from build123d import *

# Parameters (mm, degrees)
BOSS_EXTRUDE1_DEPTH = 6.35
CUT_EXTRUDE1_DEPTH  = 7.35
SKETCH4_R           = 3
CUT_EXTRUDE2_DEPTH  = 7.35


with BuildPart() as part:
    # Sketch2 → Boss-Extrude1 (new body)
    with BuildSketch(Plane.XY):
        with BuildLine():
            ThreePointArc((-100, 73.02486306), (0, 79.721425695), (100, 73.02486306))
            ThreePointArc((100, 73.02486306), (123.825, 0), (100, -73.02486306))
            ThreePointArc((100, -73.02486306), (0, -79.721425695), (-100, -73.02486306))
            ThreePointArc((-100, -73.02486306), (-123.825, 0), (-100, 73.02486306))
        make_face()
    extrude(amount=BOSS_EXTRUDE1_DEPTH)

    # Sketch3 → Cut-Extrude1 (cut, through all)
    with BuildSketch(Plane.XY.offset(6.35)):
        with BuildLine():
            Line((-61.572799723, 14.542440806), (-81.281148146, 14.542440806))
            ThreePointArc((-81.281148146, 14.542440806), (-91.5900314, 19.825101253), (-93.322799723, 31.278357963))
            ThreePointArc((-93.322799723, 31.278357963), (-87.27608067, 45.501278749), (-79.077484693, 58.602321112))
            ThreePointArc((-79.077484693, 58.602321112), (-75.119328128, 62.098990903), (-70.081085695, 63.683230851))
            ThreePointArc((-70.081085695, 63.683230851), (-59.910981492, 64.583293189), (-49.729388954, 65.342440806))
            ThreePointArc((-49.729388954, 65.342440806), (-40.200680121, 61.949526114), (-36.172799723, 52.671361338))
            Line((-36.172799723, 52.671361338), (-36.172799723, 39.942440806))
            ThreePointArc((-36.172799723, 39.942440806), (-43.612287481, 21.981928564), (-61.572799723, 14.542440806))
        make_face()
        with BuildLine():
            Line((36.172799723, -29.907559194), (36.172799723, -52.671361338))
            ThreePointArc((36.172799723, -52.671361338), (40.200680121, -61.949526114), (49.729388954, -65.342440806))
            ThreePointArc((49.729388954, -65.342440806), (59.910981492, -64.583293189), (70.081085695, -63.683230851))
            ThreePointArc((70.081085695, -63.683230851), (75.119328128, -62.098990903), (79.077484693, -58.602321112))
            ThreePointArc((79.077484693, -58.602321112), (89.8734441, -40.12785405), (96.421721635, -19.756827222))
            ThreePointArc((96.421721635, -19.756827222), (93.820577654, -9.179038283), (83.980209166, -4.507559194))
            Line((83.980209166, -4.507559194), (61.572799723, -4.507559194))
            ThreePointArc((61.572799723, -4.507559194), (43.612287481, -11.947046951), (36.172799723, -29.907559194))
        make_face()
        with BuildLine():
            Line((-61.572799723, -4.507559194), (-83.980209166, -4.507559194))
            ThreePointArc((-83.980209166, -4.507559194), (-93.820577654, -9.179038283), (-96.421721635, -19.756827222))
            ThreePointArc((-96.421721635, -19.756827222), (-89.8734441, -40.12785405), (-79.077484693, -58.602321112))
            ThreePointArc((-79.077484693, -58.602321112), (-75.119328128, -62.098990903), (-70.081085695, -63.683230851))
            ThreePointArc((-70.081085695, -63.683230851), (-59.910981492, -64.583293189), (-49.729388954, -65.342440806))
            ThreePointArc((-49.729388954, -65.342440806), (-40.200680121, -61.949526114), (-36.172799723, -52.671361338))
            Line((-36.172799723, -52.671361338), (-36.172799723, -29.907559194))
            ThreePointArc((-36.172799723, -29.907559194), (-43.612287481, -11.947046951), (-61.572799723, -4.507559194))
        make_face()
        with BuildLine():
            Line((36.172799723, 39.942440806), (36.172799723, 52.671361338))
            ThreePointArc((36.172799723, 52.671361338), (40.200680121, 61.949526114), (49.729388954, 65.342440806))
            ThreePointArc((49.729388954, 65.342440806), (59.910981492, 64.583293189), (70.081085695, 63.683230851))
            ThreePointArc((70.081085695, 63.683230851), (75.119328128, 62.098990903), (79.077484693, 58.602321112))
            ThreePointArc((79.077484693, 58.602321112), (87.27608067, 45.501278749), (93.322799723, 31.278357963))
            ThreePointArc((93.322799723, 31.278357963), (91.5900314, 19.825101253), (81.281148146, 14.542440806))
            Line((81.281148146, 14.542440806), (61.572799723, 14.542440806))
            ThreePointArc((61.572799723, 14.542440806), (43.612287481, 21.981928564), (36.172799723, 39.942440806))
        make_face()
    extrude(amount=-CUT_EXTRUDE1_DEPTH, mode=Mode.SUBTRACT)

    # Sketch4 → Cut-Extrude2 (cut, through all)
    with BuildSketch(Plane.XY.offset(6.35)):
        with Locations((-19.05, 10.998522628)):
            Circle(SKETCH4_R)
        with Locations((19.05, 10.998522628)):
            Circle(SKETCH4_R)
        with Locations((0, -21.997045256)):
            Circle(SKETCH4_R)
    extrude(amount=-CUT_EXTRUDE2_DEPTH, mode=Mode.SUBTRACT)


solid = part.part
Part model, mm, in its own coordinate system. Give positions to 0.01 mm unless a question says otherwise; leave off trailing zeros. Loops run counter-clockwise (first coordinate to the right, second up) from the corner with the lowest first, then second, coordinate; pieces in that order, holes last.
(1) Drill centre lines: line 1 along Y through (x, z) = (42.5, 4.25); line 2 along X through (y, z) = (-46, 6); line 3 along Y through (x, z) = (65, 0.5). Where is each one in solid material? Low to high.
Return value:
line 1: y = -78.52 to -63.66, -13.13 to 23.17, 63.66 to 78.52
line 2: x = -114.96 to -87.01, -36.17 to 36.17, 87.01 to 114.96
line 3: y = -76.9 to -64.15, -4.51 to 14.54, 64.15 to 76.9
(2) Band-saw the part on B-B (x = -19.05). Write the cut outline in (y, z), and give its area (3 significant figures).
Return value:
outline: (-79.48, 0) - (8, 0) - (8, 6.35) - (-79.48, 6.35) - close; (14, 0) - (79.48, 0) - (79.48, 6.35) - (14, 6.35) - close
area: 971 mm2
(3) Band-saw the part on C-C (z = 4.5). Count the separate pieces of the cut face and the enclosed holes in it, and give its area (3 significant figures).
Return value:
separate pieces: 1
enclosed holes: 7
area: 24,800 mm2
(4) Band-saw the part on A-A (x = -54.5). Write the cut outline in (y, z).
Return value:
outline: (-77.74, 0) - (-65, 0) - (-65, 6.35) - (-77.74, 6.35) - close; (-5.51, 0) - (15.55, 0) - (15.55, 6.35) - (-5.51, 6.35) - close; (65, 0) - (77.74, 0) - (77.74, 6.35) - (65, 6.35) - close
(5) Pin check, flat tips, straight feed: pin 1 (2 mm diameter, centred on y = -62.5, z = 1.5, fed in from -X); pin 2 (1.9 mm diameter, centred on x = -67.5, z = 4, fed in from +Y); pin 3 (3 mm diameter, centred on y = 48, z = 4.5, fed in from +X). Stop position of each tip, or through.
Return value:
pin 1: stops at x = -107.47
pin 2: stops at y = 76.76
pin 3: stops at x = 114.76
